Geometry: see drawing. Coordinates: mm, zero at the bounding-box minimum. Give positions to 0.01 mm unless a question says otherwise; leave off trailing zeros. Loops run counter-clockwise (first coordinate to the right, second up) from the corner with the lowest first, then second, coordinate; pieces in that order, holes last. Notation, with made-up numbers: (89.25, 2.5) - (102.25, 2.5) arc R12 ccw to (102.25, 12.5) - close; hole circle Ø8 at (40.5, 9.5). An arc over 180 degrees is marked (long way). One line per question, with ' | ' between items. Start each with the question number.
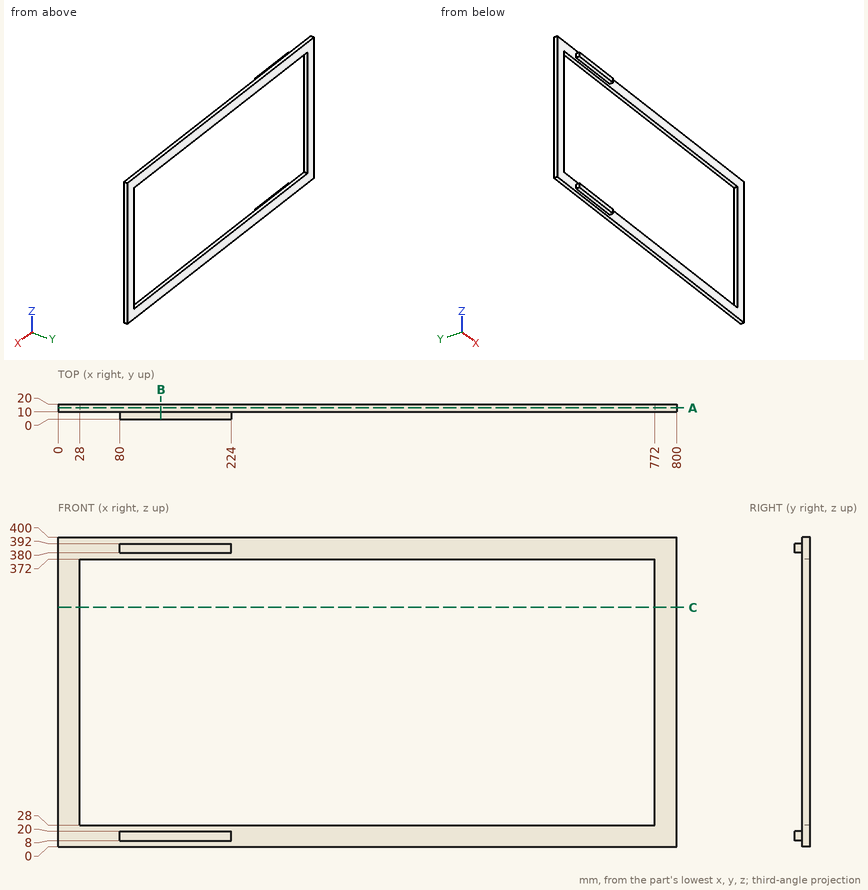
Q1. Line query: L1, parallel to Z at x = 639.5, y = 16; L2, parallel to X at y = 16.25, z = 81; L3, parallel to X at y = 2.25, z = 17. Output: solid intervals per line, ascending. Write a range as from..to.
Q2. Section A-A, the plane y = 15. Output: boundary loops of the cut face in (x, z).
Q3. Section C-C, the plane z = 309.5. Output: boundary loops of the cut face in (x, y).
Q4. First-contact query: pin 1 (5 mm diameter, centred on x = 154, y = 6, fed in from +Z); pin 2 (11 mm diameter, centred on y = 3.5, z = 15.5, fed in from +X); pin 3 (11 mm diameter, centred on x = 123.5, y = 4, fed in from -Z). Flat tips, straight axial feed; report the tip coordinate or a pass-through.
Q5. Section B-B, the plane x = 133. Output: boundary loops of the cut face in (y, z), plus the area to 3 significant figures.
Solved:
1) L1: z = 0..28, 372..400 | L2: x = 0..28, 772..800 | L3: x = 80..224
2) outline: (0, 0) - (800, 0) - (800, 400) - (0, 400) - close; hole (28, 28) - (772, 28) - (772, 372) - (28, 372) - close
3) outline: (0, 10) - (28, 10) - (28, 20) - (0, 20) - close; (772, 10) - (800, 10) - (800, 20) - (772, 20) - close
4) pin 1: stops at z = 392 | pin 2: stops at x = 224 | pin 3: stops at z = 8
5) outline: (0, 8) - (10, 8) - (10, 0) - (20, 0) - (20, 28) - (10, 28) - (10, 20) - (0, 20) - close; (0, 380) - (10, 380) - (10, 372) - (20, 372) - (20, 400) - (10, 400) - (10, 392) - (0, 392) - close | area: 800 mm²
